Drawing for the job (mm, zero at the part's lowest x, y, z). A direction names the side the tool comes from. Round coordinates to 2 decimals unless told otherwise and drop trailing zeros. Write each loop counter-clockwise with the first axis right and the second up, starting at its lowest first coordinate (ties: lowest second). Pieces come first, ordered by that corner, then holes. Notation, with made-up numbers: M -14.75,-9 L -10.75,-9 A15 ccw -10.75,4 Z; hole C -1.5,-20.5 d6. An arc over 180 degrees is marked long. Use a Markdown table: item, result.
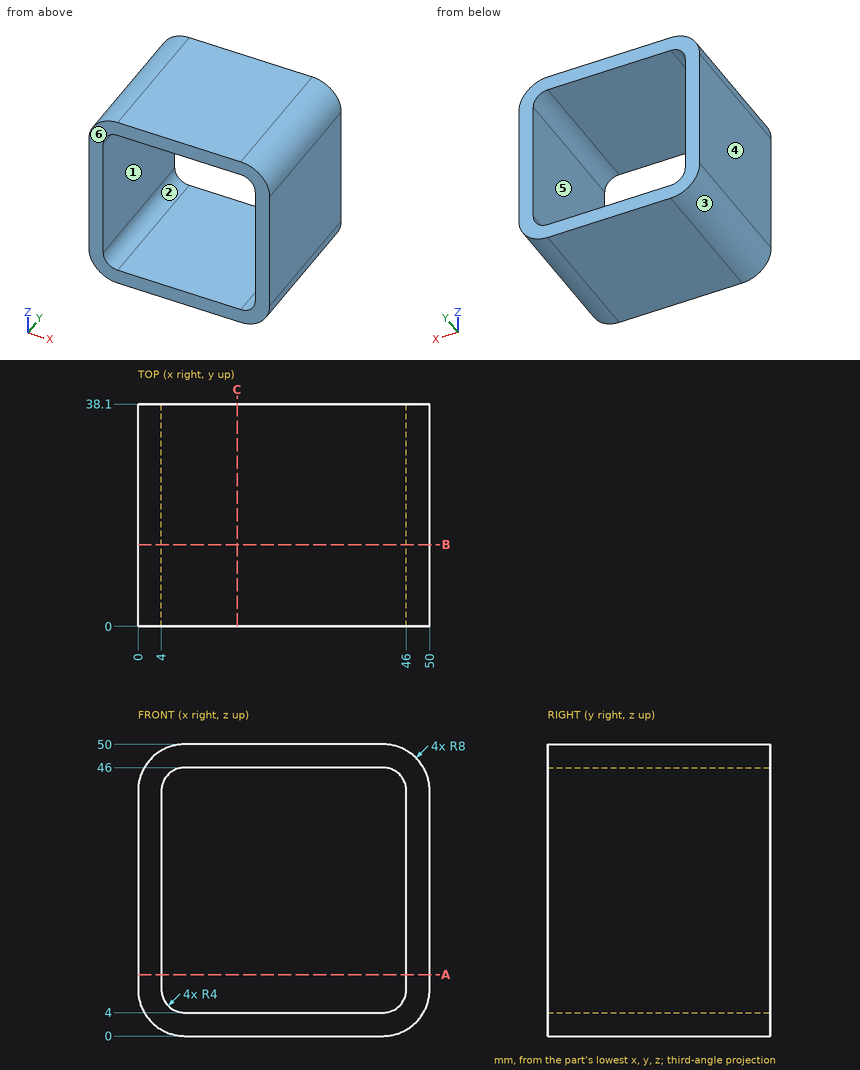
Q1. Cut at B-B on y = 14. Give the cut face in (x, z).
Response values:
| item | result |
|---|---|
| outline | M 0,8 A8 ccw 8,0 L 42,0 A8 ccw 50,8 L 50,42 A8 ccw 42,50 L 8,50 A8 ccw 0,42 Z; hole M 4,8 A4 ccw 8,4 L 42,4 A4 ccw 46,8 L 46,42 A4 ccw 42,46 L 8,46 A4 ccw 4,42 Z |
Q2. Drop a flat-ended pin along its axis: P1, Ø1, axis at x = 22, z = 44, coming from the -Y side. Give the stop position or say it passes through.
Response values:
| item | result |
|---|---|
| P1 | passes through |
Q3. Cut at A-A on z = 10.5. Give the cut face in (x, y), and give its area (3 significant figures).
Response values:
| item | result |
|---|---|
| outline | M 0,0 L 4,0 L 4,38.1 L 0,38.1 Z; M 46,0 L 50,0 L 50,38.1 L 46,38.1 Z |
| area | 305 mm2 |
Q4. Two-plate mould, pull along Z, no slides. Class the marked faces 1, 2, 3 and 4: +Z half, -Z half, draft (parallel to the pull), parting line (faces both ways), or undercut.
Response values:
| item | result |
|---|---|
| face 1 | undercut |
| face 2 | undercut |
| face 3 | -Z half |
| face 4 | draft |
Q5. Drill centre lines: L1, parallel to Z at x = 8.5, y = 22.5; L2, parallel to Z at x = 3, y = 11.5 (3 decimals). Where is each one in solid material? Low to high.
Response values:
| item | result |
|---|---|
| L1 | z = 0 to 4, 46 to 50 |
| L2 | z = 1.755 to 48.245 |
Q6. Cut at C-C on x = 17. Give the cut face in (y, z).
Response values:
| item | result |
|---|---|
| outline | M 0,0 L 38.1,0 L 38.1,4 L 0,4 Z; M 0,46 L 38.1,46 L 38.1,50 L 0,50 Z |
Q7. Which spindle directions (+Z, -Z, +X, -X, +Y, -Y) get a long thin tool onto all of the face, cutting with end or side? Do the marked faces 5 and 6. Say none if no direction does.
Response values:
| item | result |
|---|---|
| face 5 | +Y, -Y |
| face 6 | +Z, -Z, +X, -X, -Y |
